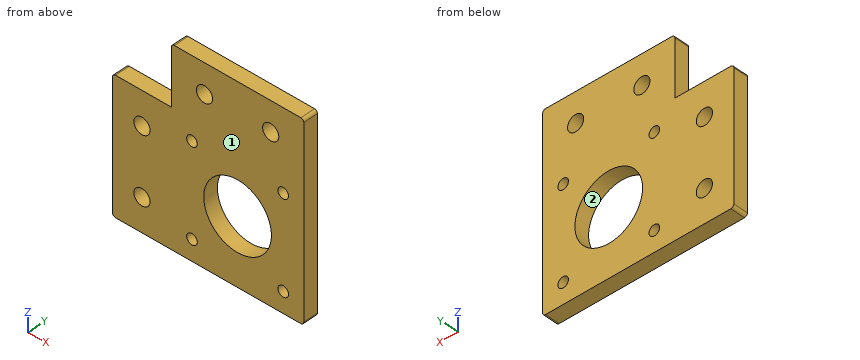
Autodesk Inventor part; units mm, degrees
ref_plane "YZ Plane" through (0, 0, 0) normal (1, 0, 0) x (0, 1, 0)
ref_plane "XZ Plane" through (0, 0, 0) normal (0, 1, 0) x (-1, 0, 0)
ref_plane "XY Plane" through (0, 0, 0) normal (0, 0, 1) x (1, 0, 0)
sketch "Sketch1" plane through (0, 0, 0) normal (0, 1, 0) x (-1, 0, 0)
  line L0 (0, 0) -> (-31, 0) construction
  line L1 (-31, 0) -> (-31, -31) construction
  line L2 (-31, -31) -> (0, -31) construction
  line L3 (0, -31) -> (0, 0) construction
  circle A0 centre (0, 0) radius 1.8
  circle A1 centre (0, -31) radius 1.8
  circle A2 centre (-31, -31) radius 1.8
  circle A3 centre (-31, 0) radius 1.8
  line L4 (-38, 7) -> (-38, -38)
  line L5 (-38, -38) -> (7, -38)
  line L6 (7, -38) -> (27, -38)
  line L7 (27, -38) -> (27, 7)
  line L8 (27, 7) -> (7, 7)
  line L9 (-38, 7) -> (-38, 27)
  line L10 (-38, 27) -> (7, 27)
  line L11 (7, 27) -> (7, 7)
  line L12 (7, 7) -> (-38, -38) construction
  line L13 (-38, 7) -> (7, -38) construction
  line L14 (17, 7) -> (17, -15.5) construction
  line L15 (7, 17) -> (-15.5, 17) construction
  line L16 (-15.5, 27) -> (-15.5, 17) construction
  line L17 (-15.5, 17) -> (-38, 17) construction
  line L18 (27, -15.5) -> (17, -15.5) construction
  line L19 (17, -15.5) -> (17, -38) construction
  circle A4 centre (17, -4.25) radius 2.75
  circle A5 centre (17, -26.75) radius 2.75
  circle A6 centre (-26.75, 17) radius 2.75
  circle A7 centre (-4.25, 17) radius 2.75
  circle A8 centre (-15.5, -15.5) radius 11.5
  dimension "d0" = 31
  dimension "d1" = 31
  dimension "d2" = 3.6
  dimension "d3" = 3.6
  dimension "d4" = 3.6
  dimension "d5" = 3.6
  dimension "d6" = 45
  dimension "d7" = 45
  dimension "d8" = 20
  dimension "d9" = 20
  dimension "d10" = 5.5
  dimension "d11" = 5.5
  dimension "d12" = 5.5
  dimension "d13" = 5.5
  dimension "d17" = 23
extrude "Extrusion1" add sketch "Sketch1" along normal blind 5
fillet "Fillet1" radius 1 5 edges at (-27, 2.5, 7) (-7, 2.5, 27) (38, 2.5, 27) (38, 2.5, -38) (-27, 2.5, -38)
equation "\"d3\" = d2"
equation "\"d4\" = d2"
equation "\"d5\" = d2"
equation "\"d11\" = d10"
equation "\"d12\" = d10"
equation "\"d13\" = d10"
properties part number "NEMA17 Stepper CornerMount" material "PC/ABS Plastic"
Source: CAD feature listing. Evaluate the final solid. Frame: model axes, mm. Face numbers are marked on the shaded views. Round coordinates to 2 decimals unless told otherwise and drop trailing zeros. Loops run counter-clockwise (first coordinate to the right, second up) from the corner with the lowest first, then second, coordinate; pieces in that order, holes last.
1. Contact query for a flat-ended pin moving along its axis: pin 1 (1.5 mm diameter, centred on x = 22.5, z = 4.5, fed in from -Y). Output: stop coordinate, or through.
2. Section query A-A on x = 31. Output: boundary loops of the cut face in (y, z).
3. Mould query, pull axis X, two halves, no side actions, for the marked faces 1 and 2. Classes: released by +X, released by -X, zero draft, split by the parting line, or undercut.
4. Section query D-D on x = 15.5. Output: boundary loops of the cut face in (y, z), and give its area (3 significant figures).
5. Ray query, L1, parallel to Z at x = 0, y = 1.4; L2, parallel to Z at x = -19.5, y = 1.95; L3, parallel to X at y = 1.85, z = -15. Return the intervals inside material, ascending.
6. Section query C-C on y = 2.9. Give the number of separate pieces and of enclosed holes in the cut face, and give its area (3 significant figures).
7. Section query B-B on z = -31. Output: boundary loops of the cut face in (x, y).
Answers below:
1. pin 1: stops at y = 0
2. outline: (0, -38) - (5, -38) - (5, -32.8) - (0, -32.8) - close; (0, -29.2) - (5, -29.2) - (5, -1.8) - (0, -1.8) - close; (0, 1.8) - (5, 1.8) - (5, 27) - (0, 27) - close
3. face 1: zero draft
3. face 2: undercut
4. outline: (0, -38) - (5, -38) - (5, -27) - (0, -27) - close; (0, -4) - (5, -4) - (5, 27) - (0, 27) - close
4. area: 210 mm2
5. L1: z = -38 to -32.8, -29.2 to -1.8, 1.8 to 27
5. L2: z = -38 to -27.9, -25.6 to -5.4, -3.1 to 7
5. L3: x = -27 to 4.01, 26.99 to 38
6. separate pieces: 1
6. enclosed holes: 9
6. area: 3,270 mm2
7. outline: (-27, 0) - (-1.8, 0) - (-1.8, 5) - (-27, 5) - close; (1.8, 0) - (29.2, 0) - (29.2, 5) - (1.8, 5) - close; (32.8, 0) - (38, 0) - (38, 5) - (32.8, 5) - close
